Model file for the job. Use its own axes, mm. Round coordinates to 2 decimals unless told otherwise and drop trailing zeros. Order: outer loops, then holes, each group sorted by start corner. A loop starts at its lowest first (then second) coordinate and runs counter-clockwise, first axis right, second up. Notation, with made-up numbers: (-2.75, 75.25) -> (47.25, 75.25) arc R19 cw to (47.25, 96.25) -> close; hole circle Ø4 at (3.25, 59). An arc over 180 degrees is marked (long way). Answer as CSV lines item,"result".
```python
from build123d import *

# Parameters (mm, degrees)
BOSS_EXTRUDE1_DEPTH = 3.175
CUT_EXTRUDE1_DEPTH  = 135.915478092


with BuildPart() as part:
    # Sketch1 → Boss-Extrude1 (new body)
    with BuildSketch(Plane.XY):
        with BuildLine():
            Line((-101.484623167, 0), (-112.493407504, 6.355924601))
            ThreePointArc((-112.493407504, 6.355924601), (0, 74.413297682), (112.493407504, 6.355924601))
            Line((112.493407504, 6.355924601), (101.484623167, 0))
            ThreePointArc((101.484623167, 0), (0, 61.713297682), (-101.484623167, 0))
        make_face()
    extrude(amount=BOSS_EXTRUDE1_DEPTH)

    # Sketch2 → Cut-Extrude1 (cut, symmetric)
    with BuildSketch(Plane.XY.offset(3.175)):
        with BuildLine():
            Line((112.493407504, 6.355924601), (106.989015336, 3.1779623))
            Line((106.989015336, 3.1779623), (105.401515336, 5.927592957))
            Line((105.401515336, 5.927592957), (110.984177534, 9.15074448))
            ThreePointArc((110.984177534, 9.15074448), (111.747530211, 7.758052979), (112.493407504, 6.355924601))
        make_face()
    cut_extrude1 = extrude(amount=CUT_EXTRUDE1_DEPTH, both=True, mode=Mode.SUBTRACT)

    # Mirror1: Cut-Extrude1 across plane
    add(cut_extrude1.mirror(Plane(origin=(0, 0, 0), x_dir=(0, 0, 1), z_dir=(1, 0, 0))), mode=Mode.SUBTRACT)


solid = part.part
```
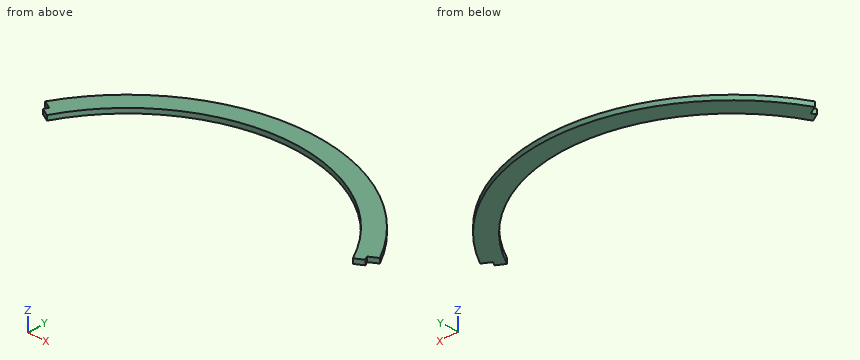
Q1. Saw through at D-D (x = -23.5). Write the cut outline in (y, z) (3 decimals).
Checks:
outline,"(59.271, 0) -> (72.22, 0) -> (72.22, 3.175) -> (59.271, 3.175) -> close"
Q2. Saw through at B-B (z = 1.85). Write the cut outline in (x, y).
Checks:
outline,"(-110.98, 9.15) -> (-105.4, 5.93) -> (-106.99, 3.18) -> (-101.48, 0) arc R114.3 cw to (101.48, 0) -> (106.99, 3.18) -> (105.4, 5.93) -> (110.98, 9.15) arc R127 ccw to start"
Q3. Saw through at A-A (y = 45.5). Write the cut outline in (x, z) (3 decimals).
Checks:
outline,"(-80.672, 0) -> (-58.681, 0) -> (-58.681, 3.175) -> (-80.672, 3.175) -> close; (58.681, 0) -> (80.672, 0) -> (80.672, 3.175) -> (58.681, 3.175) -> close"
Q4. Wall check: L1, parallel to X at y = 28, z = 2.7; L2, parallel to X at y = 18, z = 2.5; L3, parallel to Y at x = -80, z = 0.65. Give the ranges that are in metal, low to high. Write a range as [from, to].
Checks:
L1,"[-98.16, -81.06], [81.06, 98.16]"
L2,"[-105.58, -89.9], [89.9, 105.58]"
L3,"[29.05, 46.05]"
Q5. Saw through at C-C (y = 12). Write the cut outline in (x, z) (3 decimals).
Checks:
outline,"(-109.351, 0) -> (-94.303, 0) -> (-94.303, 3.175) -> (-109.351, 3.175) -> close; (94.303, 0) -> (109.351, 0) -> (109.351, 3.175) -> (94.303, 3.175) -> close"
Q6. Flat gauge pins, fed straight in: pin 1 (1.5 mm diameter, centred on y = 63.5, z = 2, fed in from +X); pin 2 (10 mm diameter, centred on x = -53.5, y = 60.5, fed in from -Z); pin 3 (1 mm diameter, centred on x = -48.5, z = 2, fed in from +Y). Where does each tip first touch, or does it go through?
Checks:
pin 1,"x = 53.16"
pin 2,"z = 0"
pin 3,"y = 64.99"
